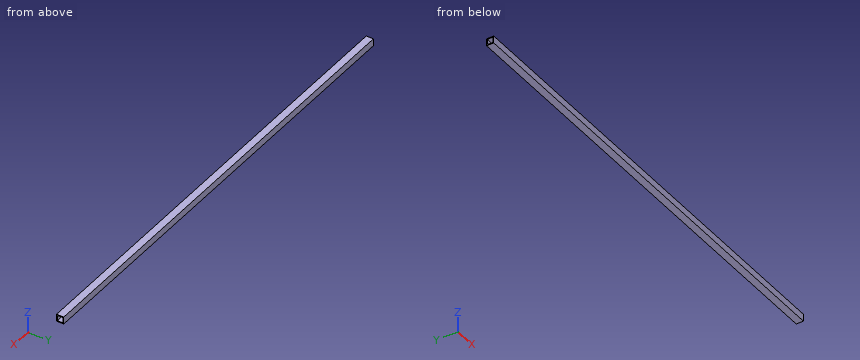
Autodesk Inventor part; units mm, degrees
ref_plane "YZ Plane" through (0, 0, 0) normal (1, 0, 0) x (0, 1, 0)
ref_plane "XZ Plane" through (0, 0, 0) normal (0, 1, 0) x (-1, 0, 0)
ref_plane "XY Plane" through (0, 0, 0) normal (0, 0, 1) x (1, 0, 0)
sketch "Sketch1" plane through (0, 0, 0) normal (1, 0, 0) x (0, 1, 0)
  circle A0 centre (0, 0) radius 10
  dimension "d0" = 20
extrude "Extrusion1" add sketch "Sketch1" against normal blind 1300
sketch "Sketch2" plane through (0, 0, 0) normal (1, 0, 0) x (0, 0, -1)
  circle A0 centre (0, 0) radius 10
  circle A1 centre (0, 0) radius 7.5
  dimension "d5" = 15
extrude "Extrusion2" cut sketch "Sketch2" against normal blind 1300 contours A1
sketch "Sketch4" plane through (0, 0, 0) normal (1, 0, 0) x (0, 0, -1)
  circle A0 centre (0, 0) radius 10
  line L0 (0, -10) -> (10, -10)
  line L1 (10, -10) -> (10, 0)
  line L2 (10, 10) -> (-10, 10)
  line L3 (-10, 10) -> (-10, 0)
  line L4 (10, 0) -> (10, 10)
  line L5 (-10, 0) -> (-10, -10)
  line L6 (0, -10) -> (-10, -10)
extrude "Extrusion3" add sketch "Sketch4" against normal blind 1300 contours L3 L2 A0 | A0 L6 L5 | A0 L1 L0 | L2 L4 A0
sketch "Sketch5" plane through (0, 0, 0) normal (1, 0, 0) x (0, 0, -1)
  circle A0 centre (0, 0) radius 7.5
  line L0 (7.5, 0) -> (7.5, -7.5)
  line L1 (7.5, -7.5) -> (0, -7.5)
  line L2 (0, -7.5) -> (-7.5, -7.5)
  line L3 (-10, -10) -> (10, -10)
  line L4 (-7.5, 0) -> (-7.5, -7.5)
  line L5 (-7.5, 0) -> (-7.5, 7.5)
  line L6 (0, 7.5) -> (-7.5, 7.5)
  line L7 (0, 7.5) -> (7.5, 7.5)
  line L8 (7.5, 0) -> (7.5, 7.5)
extrude "Extrusion4" cut sketch "Sketch5" against normal blind 1300 contours L0 L1 A0 | A0 L7 L8 | A0 L5 L6 | L2 L4 A0
properties part number "rail"
Read the model definition and answer for the solid it produces. Units are mm, in the model's axes. Give positions to 0.01 mm unless a question says otherwise; leave off trailing zeros. Write each loop counter-clockwise with the first axis right and the second up, starting at its lowest first coordinate (ties: lowest second). Pieces come first, ordered by that corner, then holes. Notation, with made-up numbers: (66.25, 69.25) - (108.25, 69.25) arc R3 ccw to (108.25, 74.25) - close; hole circle Ø7 at (11.5, 73). An arc over 180 degrees is marked (long way). Write item = value, one per line. Start each with the question number.
Item 1: Find section A-A (y = -0.5). Give the vertices of the cut face in (x, z).
Item 2: Find the intervals of material crossed by probe 1 along Y at (x, z) = (-552.5, 3), in increasing order. Write a range as [from, to].
Item 3: Find section C-C (x = -472.5). Give the vertices of the cut face in (y, z), then the cut area to 3 significant figures.
Response:
q1.outline = (-1300, -10) - (0, -10) - (0, -7.5) - (-1300, -7.5) - close; (-1300, 7.5) - (0, 7.5) - (0, 10) - (-1300, 10) - close
q2.probe_1 = [-10, -7.5], [7.5, 10]
q3.outline = (-10, -10) - (10, -10) - (10, 10) - (-10, 10) - close; hole (-7.5, -7.5) - (7.5, -7.5) - (7.5, 7.5) - (-7.5, 7.5) - close
q3.area = 175 mm²
